Read the model definition and answer for the solid it produces. Units are mm, in the model's axes. A direction names the side the tool comes from. Round coordinates to 2 decimals unless told otherwise and drop trailing zeros. Write each loop counter-clockwise with the first axis right and the second up, starting at its lowest first coordinate (ties: lowest second). Pieces come first, ordered by that corner, then holes. Notation, with made-up numbers: (81.5, 60) -> (116.5, 60) arc R24 ccw to (116.5, 91) -> close; hole circle Ø5 at (-15.75, 69). An arc over 180 degrees is marked (long way). Return JSON: item names as keys, results as strings.
from build123d import *

# Parameters (mm, degrees)
F0_W     = 182
F0_H     = 53
F1_DEPTH = 200
F2_DEPTH = 80
F3_W     = 182
F3_H     = 53
F4_DEPTH = 5
F0_W_2   = 202
F0_H_2   = 131
F5_DEPTH = 5


with BuildPart() as f1:
    # F0 (on Top) → F1 (new body)
    with BuildSketch(Plane.XY):
        Polygon((81.89805, -3.570612), (-100.10195, -3.570612), (-105.10195, -3.570612), (-105.10195, -66.570612), (86.89805, -66.570612), (86.89805, -3.570612), align=None)
        with Locations((-9.10195, -35.070612)):
            Rectangle(F0_W, F0_H, mode=Mode.SUBTRACT)
    extrude(amount=-F1_DEPTH)

    # F0 (on Top) → F2 (join)
    with BuildSketch(Plane.XY):
        Polygon((-100.10195, -3.570612), (-100.10195, 49.429388), (81.89805, 49.429388), (81.89805, -3.570612), (86.89805, -3.570612), (86.89805, 54.429388), (-105.10195, 54.429388), (-105.10195, -3.570612), align=None)
    extrude(amount=-F2_DEPTH)

    # F3 (on face) → F4 (join)
    with BuildSketch(Plane(origin=(0, 0, -200), x_dir=(1, 0, 0), z_dir=(0, 0, -1))):
        with Locations((-9.10195, 35.070612)):
            Rectangle(F3_W, F3_H)
    extrude(amount=-F4_DEPTH)

    # F0 (on Top) → F5 (join)
    with BuildSketch(Plane.XY):
        with Locations((-9.10195, -6.070612)):
            Rectangle(F0_W_2, F0_H_2)
        Polygon((-105.10195, -66.570612), (-105.10195, -3.570612), (-105.10195, 54.429388), (86.89805, 54.429388), (86.89805, -3.570612), (86.89805, -66.570612), align=None, mode=Mode.SUBTRACT)
    extrude(amount=-F5_DEPTH)


solid = f1.part
Item 1: Straight lines are drawn through the part: L1, parallel to Y at x = 39.5, z = -28.5; L2, parallel to X at y = -47.5, z = -167; L3, parallel to Y at x = 21.5, z = -176.5. For each, find the intervals that lie inside material, in ascending order. Write a range as [from, to].
Worked answers:
{"L1": "y = [-66.57, -61.57], [-8.57, -3.57], [49.43, 54.43]", "L2": "x = [-105.1, -100.1], [81.9, 86.9]", "L3": "y = [-66.57, -61.57], [-8.57, -3.57]"}
Item 2: Flat-ended cylindrical pins translate along their axes: pin 1 (10 mm diameter, centred on x = -36, z = -80.5, fed in from -Y); pin 2 (16 mm diameter, centred on x = -18.5, y = -23.5, fed in from +Z); pin 3 (16 mm diameter, centred on y = 33, z = -33.5, fed in from +X). Find the tip coordinate at first contact, or state that the pin passes through.
Worked answers:
{"pin 1": "stops at y = -66.57", "pin 2": "stops at z = -195", "pin 3": "stops at x = 86.9"}
Item 3: Section A-A (y = 32) is taken. Give the vertices of the cut face in (x, z).
Worked answers:
{"outline": "(-110.1, -5) -> (-105.1, -5) -> (-105.1, -80) -> (-100.1, -80) -> (-100.1, 0) -> (-110.1, 0) -> close; (81.9, -80) -> (86.9, -80) -> (86.9, -5) -> (91.9, -5) -> (91.9, 0) -> (81.9, 0) -> close"}
Item 4: Section C-C (x = 4.5) is taken. Give the vertices of the cut face in (y, z), then the cut area to 4 significant figures.
Worked answers:
{"outline": "(-71.57, -5) -> (-66.57, -5) -> (-66.57, -200) -> (-3.57, -200) -> (-3.57, 0) -> (-8.57, 0) -> (-8.57, -195) -> (-61.57, -195) -> (-61.57, 0) -> (-71.57, 0) -> close; (49.43, -80) -> (54.43, -80) -> (54.43, -5) -> (59.43, -5) -> (59.43, 0) -> (49.43, 0) -> close", "area": "2,715 mm2"}
Item 5: Section D-D (z = -168.5) is taken. Give the vertices of the cut face in (x, y), then the cut area to 3 significant figures.
Worked answers:
{"outline": "(-105.1, -66.57) -> (86.9, -66.57) -> (86.9, -3.57) -> (-105.1, -3.57) -> close; hole (-100.1, -61.57) -> (81.9, -61.57) -> (81.9, -8.57) -> (-100.1, -8.57) -> close", "area": "2,450 mm2"}
Item 6: For a pull along X with two mould halves and no side action, classify faces 4 (the flat face through (86.898, -20, -79)), 5 (the flat face through (-33, -5, 0)), 6 (the flat face through (81.898, -35, -96)) as released by +X, released by -X, zero draft, split by the parting line, or undercut.
Worked answers:
{"face 4": "released by +X", "face 5": "zero draft", "face 6": "undercut"}
Item 7: Section B-B (z = -13) is taken. Give the vertices of the cut face in (x, y), then the cut area to 3 significant figures.
Worked answers:
{"outline": "(-105.1, -66.57) -> (86.9, -66.57) -> (86.9, 54.43) -> (-105.1, 54.43) -> close; hole (-100.1, -61.57) -> (81.9, -61.57) -> (81.9, -8.57) -> (-100.1, -8.57) -> close; hole (-100.1, -3.57) -> (81.9, -3.57) -> (81.9, 49.43) -> (-100.1, 49.43) -> close", "area": "3,940 mm2"}
Item 8: A tool of negligible diameter and unlimited length cuts with its end or side. For faces 1 (the flat face through (-100.102, -35, -96)), 2 (the flat face through (-8, 54.429, -42)), 3 (the flat face through (-10, -66.571, -101)), from which of +Z, -Z, +X, -X, +Y, -Y can it reach the whole face along a straight path? Write none if from no direction.
Worked answers:
{"face 1": "+Z", "face 2": "-Z, +X, -X, +Y", "face 3": "-Z, +X, -X, -Y"}
